The model under review builds one solid part; all positions refer to its coordinate system, in mm. A direction names the side the tool comes from. Give positions to 0.01 mm unless a question says otherwise; leave off trailing zeros. Loops run counter-clockwise (first coordinate to the right, second up) from the corner with the lowest first, then second, coordinate; pieces in that order, holes last. Notation, with made-up numbers: M -4,6 L 40,6 A5 ccw 40,15 Z; hole C 50,-30 d7. An arc over 180 degrees is marked long. One line per item, written item: value. Start each with the question number.
Q1. We need section C-C on z = -5.75. Write out the cut boundary in (x, y).
Q2. We need section B-B on x = 10. Write out the cut boundary in (y, z).
Q3. To check wall thickness, follow line 1 along X through (y, z) = (8, 4.5); line 2 along X through (y, z) = (21.5, -6). State the ranges of each line that lie inside material, in increasing order. Write a range as from..to.
Q4. We need section A-A on z = 3.75. Write out the cut boundary in (x, y), plus the area to 3 significant figures.
Q5. Mouldability with a two-part tool opening along X and no side actions: class faces 6 (the face through (21, 26, 11)), 7 (the face through (23.93, 11.324, 10.493)), 8 (the face through (4.9, 22.21, -9.14)) as released by +X, released by -X, zero draft, split by the parting line, or undercut.
Q6. For pin 1 (6 mm diameter, centred on y = 23, z = -2.5, fed in from -X); pin 2 (1.5 mm diameter, centred on x = 25.5, y = 39.5, fed in from -Z); pin 3 (2.5 mm diameter, centred on x = 28.5, z = 3.5, fed in from -Y), all flat-tipped, find the tip position at first contact; note any pin that passes through.
Q7. For faces 1 (the face through (21.15, 11.08, 10.49)), 2 (the face through (4, 22, -1)), 3 (the face through (0, 22, 6)), 4 (the face through (28.76, 11.34, 10.49)), 5 (the face through (20, 42.5, 2)), list the 3-axis set-ups (+Z, -Z, +X, -X, +Y, -Y) from which the entire face can be reached by the end or side of a thin tool; tool diameter is ignored.
Q8. We need section D-D on x = 5.5. Write out the cut boundary in (y, z), plus the area to 3 significant figures.
```python
from build123d import *

# Parameters (mm, degrees)
ESQUISSE2_W             = 44
ESQUISSE2_H             = 44
BOSS_EXTRU_1_DEPTH      = 10
ESQUISSE3_W             = 36
ESQUISSE3_H             = 36
BOSS_EXTRU_2_DEPTH      = 10
ESQUISSE4_W             = 42.5
ESQUISSE4_H             = 42.5
ESQUISSE4_W_2           = 36
ESQUISSE4_H_2           = 36
ENL_V_MAT_EXTRU_1_DEPTH = 5
CONG_1_R                = 3
CONG_2_R                = 2
BOSS_EXTRU_4_DEPTH      = 1


with BuildPart() as part:
    # Esquisse2 → Boss.-Extru.1 (new body)
    with BuildSketch(Plane.XY):
        with Locations((22, 22)):
            Rectangle(ESQUISSE2_W, ESQUISSE2_H)
    extrude(amount=BOSS_EXTRU_1_DEPTH)

    # Esquisse3 → Boss.-Extru.2 (add)
    with BuildSketch(Plane(origin=(0, 0, 0), x_dir=(-1, 0, 0), z_dir=(0, 0, -1))):
        with Locations((-22, 22)):
            Rectangle(ESQUISSE3_W, ESQUISSE3_H)
    extrude(amount=BOSS_EXTRU_2_DEPTH)

    # Esquisse4 → Enlèv. mat.-Extru.1 (cut)
    with BuildSketch(Plane(origin=(0, 0, 0), x_dir=(-1, 0, 0), z_dir=(0, 0, -1))):
        with Locations((-21.25, 21.25)):
            Rectangle(ESQUISSE4_W, ESQUISSE4_H)
        with Locations((-22, 22)):
            Rectangle(ESQUISSE4_W_2, ESQUISSE4_H_2, mode=Mode.SUBTRACT)
    extrude(amount=-ENL_V_MAT_EXTRU_1_DEPTH, mode=Mode.SUBTRACT)

    # Congé1
    cong_1_edges = [part.edges().sort_by_distance(p)[0] for p in [
        (22, 40, -10),
        (4, 22, -10),
        (22, 4, -10),
        (40, 22, -10),
        (44, 0, 5),
        (44, 44, 5),
        (0, 0, 7.5),
        (0, 44, 5),
        (4, 4, -2.5),
        (4, 40, -2.5),
        (40, 4, -2.5),
        (40, 40, -2.5),
        (42.5, 42.5, 2.5),
    ]]
    fillet(cong_1_edges, radius=CONG_1_R)

    # Congé2
    cong_2_edges = [part.edges().sort_by_distance(p)[0] for p in [
        (44, 22, 10),
        (22, 0, 10),
        (0, 22, 10),
        (22, 44, 10),
        (0.878679656, 43.121320344, 10),
        (0.878679656, 0.878679656, 10),
        (43.121320344, 43.121320344, 10),
        (43.121320344, 0.878679656, 10),
    ]]
    fillet(cong_2_edges, radius=CONG_2_R)

    # Esquisse7 → Boss.-Extru.4 (add)
    with BuildSketch(Plane.XY.offset(10)):
        with BuildLine():
            Line((15.374098957, 17.346843443), (18.030348957, 14.221843443))
            add(Edge.make_bspline(
                [(18.030348957, 14.221843443), (17.301182291, 14.32601011), (16.565114838, 14.389890267), (15.842848957, 14.534343443), (15.423010802, 14.618311074), (14.838115665, 15.028795794), (14.436598957, 15.315593443), (12.049681404, 17.020534553), (11.595795075, 19.293760446), (11.936598957, 22.190593443), (12.054157826, 23.189843826), (13.69238751, 25.196381996), (14.436598957, 25.940593443)],
                knots=[0, 0, 0, 0, 1, 1, 1, 2, 2, 2, 3, 3, 3, 4, 4, 4, 4], degree=3))
            Line((14.436598957, 25.940593443), (15.06939707, 26.573391556))
            Line((15.06939707, 26.573391556), (14.905348957, 25.784343443))
            add(Edge.make_bspline(
                [(14.905348957, 25.784343443), (14.590446041, 23.265120116), (14.091309116, 20.570212966), (14.905348957, 18.128093443), (15.001385879, 17.839982679), (15.278062036, 17.634954207), (15.374098957, 17.346843443)],
                knots=[0, 0, 0, 0, 1, 1, 1, 2, 2, 2, 2], degree=3))
        make_face()
        with BuildLine():
            Line((30.686598957, 11.878093443), (26.780348957, 10.784343443))
            Line((26.780348957, 10.784343443), (20.999098957, 11.878093443))
            Line((20.999098957, 11.878093443), (29.124098957, 13.909343443))
            ThreePointArc((29.124098957, 13.909343443), (30.444920086, 13.308773157), (30.686598957, 11.878093443))
        make_face()
        with BuildLine():
            Line((18.811598957, 7.971843443), (14.280348957, 5.471843443))
            add(Edge.make_bspline(
                [(14.280348957, 5.471843443), (14.280348957, 7.772797666), (14.593726557, 7.189715843), (13.342848957, 8.440593443)],
                knots=[0, 0, 0, 0, 1, 1, 1, 1], degree=3))
            add(Edge.make_bspline(
                [(13.342848957, 8.440593443), (13.394932291, 8.54476011), (13.404330032, 8.685401354), (13.499098957, 8.753093443), (13.783405732, 8.956169711), (14.089133052, 9.185268084), (14.436598957, 9.221843443), (16.134694919, 9.400590386), (17.384797269, 8.685244287), (18.811598957, 7.971843443)],
                knots=[0, 0, 0, 0, 1, 1, 1, 2, 2, 2, 3, 3, 3, 3], degree=3))
        make_face()
        with BuildLine():
            Line((13.200641117, 12.506283222), (29.317230938, 9.618393711))
            ThreePointArc((29.317230938, 9.618393711), (28.067553161, 8.724486443), (28.200641117, 7.193783222))
            Line((28.200641117, 7.193783222), (12.575641117, 10.631283222))
            ThreePointArc((12.575641117, 10.631283222), (12.499815902, 11.698224961), (13.200641117, 12.506283222))
        make_face()
        with BuildLine():
            add(Edge.make_bspline(
                [(20.999098957, 15.315593443), (20.827145061, 14.799731755), (21.046210645, 13.925047339), (20.530348957, 13.753093443), (20.153128088, 13.627353153), (20.137873233, 14.301819167), (20.061598957, 14.378093443), (16.567694762, 17.871997638), (14.613515541, 21.933204334), (16.467848957, 26.878093443), (17.971713728, 30.888399498), (21.846423142, 33.698659479), (22.249098957, 38.128093443)],
                knots=[4, 4, 4, 4, 5, 5, 5, 6, 6, 6, 7, 7, 7, 8, 8, 8, 8], degree=3))
            add(Edge.make_bspline(
                [(22.249098957, 38.128093443), (23.024720103, 37.74028287), (26.549972992, 30.317022339), (26.624098957, 29.378093443), (26.824723104, 26.836854256), (26.793735434, 25.141457588), (26.311598957, 22.971843443), (25.843661476, 20.866124777), (23.763276375, 19.341691827), (22.561598957, 17.659343443), (22.093633816, 17.004192245), (21.257183639, 16.089847489), (20.999098957, 15.315593443)],
                knots=[0, 0, 0, 0, 1, 1, 1, 2, 2, 2, 3, 3, 3, 4, 4, 4, 4], degree=3))
        make_face()
        with BuildLine():
            add(Edge.make_bspline(
                [(22.874098957, 14.378093443), (22.776875457, 14.340699789), (22.561598957, 14.273926776), (22.561598957, 14.378093443), (22.561598957, 17.724570677), (25.385181625, 19.244008778), (26.780348957, 22.034343443), (28.269529967, 25.012705463), (27.627114524, 26.898375507), (27.405348957, 30.003093443)],
                knots=[3, 3, 3, 3, 4, 4, 4, 5, 5, 5, 6, 6, 6, 6], degree=3))
            add(Edge.make_bspline(
                [(27.405348957, 30.003093443), (30.439237099, 28.486149372), (31.410808057, 20.585108609), (29.749098957, 17.815593443), (28.578255605, 15.864187855), (26.718288261, 15.58655694), (24.749098957, 15.003093443), (24.117435238, 14.815933822), (23.488994366, 14.614591677), (22.874098957, 14.378093443)],
                knots=[0, 0, 0, 0, 1, 1, 1, 2, 2, 2, 3, 3, 3, 3], degree=3))
        make_face()
        with BuildLine():
            add(Edge.make_bspline(
                [(13.825641117, 6.383595142), (13.664946359, 4.294397314), (12.835062605, 4.491118619), (11.307669526, 4.983380758)],
                knots=[1, 1, 1, 1, 2, 2, 2, 2], degree=3))
            add(Edge.make_bspline(
                [(11.307669526, 4.983380758), (10.888236852, 8.443524348), (13.995704046, 8.594588879), (13.825641117, 6.383595142)],
                knots=[0, 0, 0, 0, 1, 1, 1, 1], degree=3))
        make_face()
        with BuildLine():
            add(Edge.make_bspline(
                [(30.312986898, 9.093826211), (32.34922339, 8.599547626), (32.02172038, 7.812052803), (31.290447284, 6.383595142)],
                knots=[1, 1, 1, 1, 2, 2, 2, 2], degree=3))
            add(Edge.make_bspline(
                [(31.290447284, 6.383595142), (27.807867011, 6.525553152), (28.158042034, 9.616920214), (30.312986898, 9.093826211)],
                knots=[0, 0, 0, 0, 1, 1, 1, 1], degree=3))
        make_face()
    extrude(amount=BOSS_EXTRU_4_DEPTH)


solid = part.part
```
Solved:
1. outline: M 4,7 A3 ccw 7,4 L 37,4 A3 ccw 40,7 L 40,37 A3 ccw 37,40 L 7,40 A3 ccw 4,37 Z
2. outline: M 0,5 L 4,5 L 4,-7 A3 ccw 7,-10 L 37,-10 A3 ccw 40,-7 L 40,5 L 42.5,5 L 42.5,0 L 44,0 L 44,8 A2 ccw 42,10 L 2,10 A2 ccw 0,8 Z
3. line 1: 4..40, 42.5..44
3. line 2: 4..40
4. outline: M 0.4,42.5 L 39.5,42.5 A3 cw 42.5,39.5 L 42.5,0.4 A3 ccw 44,3 L 44,41 A3 ccw 41,44 L 3,44 A3 ccw Z; M 4,7 A3 ccw 7,4 L 37,4 A3 ccw 40,7 L 40,37 A3 ccw 37,40 L 7,40 A3 ccw 4,37 Z
4. area: 1,410 mm2
5. face 6: zero draft
5. face 7: undercut
5. face 8: released by -X
6. pin 1: x = 4
6. pin 2: z = -9.44
6. pin 3: y = 4
7. face 1: +Z
7. face 2: -Z, -X, -Y
7. face 3: +Z, -Z, -X, +Y, -Y
7. face 4: +Z, +X
7. face 5: -Z, -X
8. outline: M 0,5 L 4.4,5 L 4.4,-7 A2.6 ccw 7,-9.6 L 37,-9.6 A2.6 ccw 39.6,-7 L 39.6,5 L 42.5,5 L 42.5,0 L 44,0 L 44,8 A2 ccw 42,10 L 2,10 A2 ccw 0,8 Z
8. area: 737 mm2
